from build123d import *

# Parameters (mm, degrees)
BOSS_EXTRUDE1_DEPTH = 1.5875
FILLET1_R           = 2.54
CUT_EXTRUDE1_DEPTH  = 7.62


with BuildPart() as part:
    # Sketch2 → Boss-Extrude1 (new body, symmetric)
    with BuildSketch(Plane.XY):
        with BuildLine():
            add(Edge.make_bspline(
                [(825.5, 263.72872798), (833.004293944, 262.763036085), (840.535916247, 261.846014478), (848.126574562, 260.964164828), (892.90639318, 255.945629274), (937.686211733, 251.779150949), (973.452075064, 248.227669425), (1071.946672141, 239.051054038), (1170.441269319, 229.731506738), (1231.791940344, 224.503945813), (1324.899336146, 216.790627817), (1418.006730935, 209.040117978), (1449.742935921, 206.361809936), (1636.928606778, 190.521130342), (1824.114277635, 175.409157235), (1979.966947376, 164.299650253), (2156.268639429, 150.414433314), (2332.570330468, 133.857216402), (2354.212983157, 131.78508222), (2394.341467798, 127.847039259), (2434.469952439, 123.717187755), (2453.57670361, 121.704562273), (2472.669581058, 119.647220503), (2491.74, 117.547195763)],
                knots=[78.681340958, 78.681340958, 78.681340958, 78.681340958, 78.681340958, 78.681340958, 82.46579272, 82.46579272, 82.46579272, 100.7932901, 100.7932901, 100.7932901, 131.0989539, 131.0989539, 131.0989539, 146.7691983, 146.7691983, 146.7691983, 223.5339586, 223.5339586, 223.5339586, 233.9431167, 233.9431167, 233.9431167, 243.40815085, 243.40815085, 243.40815085, 243.40815085, 243.40815085, 243.40815085], degree=5))
            Line((825.5, 263.72872798), (825.5, 248.364439806))
            add(Edge.make_bspline(
                [(825.5, 248.364439806), (827.20768691, 248.14708351), (833.784664511, 247.321927102), (845.28106727, 245.953419483), (860.086531547, 244.295598067), (879.830703434, 242.186646028), (904.369967092, 239.698279806), (933.571022669, 236.832150625), (962.642718041, 234.023667741), (991.762593943, 231.241975908), (1021.072010315, 228.475862291), (1060.376437315, 224.796956681), (1109.513015577, 220.184378862), (1168.511190361, 214.817071985), (1227.500129793, 209.662054042), (1306.133167947, 203.021178328), (1404.361477105, 194.920725932), (1522.239851071, 184.918066624), (1640.182856491, 175.167007786), (1758.165352567, 165.757639485), (1876.155384769, 156.590937079), (1994.08749188, 147.453250142), (2092.268692061, 139.624216053), (2170.748029042, 133.079656729), (2219.771730977, 128.842227836), (2258.983988247, 125.347211495), (2288.379457536, 122.670854497), (2317.812243116, 119.931729386), (2347.551509172, 117.100365283), (2377.159899727, 114.21011853), (2406.469653851, 111.26896801), (2435.81832606, 108.240091266), (2464.242715806, 105.222889554), (2482.876892709, 103.192325927), (2491.74, 102.214848055)],
                knots=[78.875303138, 78.875303138, 78.875303138, 78.875303138, 79.386176103, 80.841530691, 82.29688528, 83.752239868, 86.662949044, 89.57365822, 92.484367397, 95.395076573, 98.305785749, 101.216494926, 107.037913278, 112.859331631, 118.680749984, 124.502168336, 136.145005042, 147.787841747, 159.430678452, 171.073515158, 182.716351863, 194.359188568, 206.002025273, 211.823443626, 217.644861979, 220.555571155, 223.466280331, 226.376989508, 229.287698684, 232.19840786, 235.109117037, 238.019826213, 240.930535389, 243.57402126, 243.57402126, 243.57402126, 243.57402126], degree=3))
            Line((2491.74, 102.214848055), (2491.74, 117.547195763))
        make_face()
    extrude(amount=BOSS_EXTRUDE1_DEPTH, both=True)

    # Fillet1
    fillet1_edges = [part.edges().sort_by_distance(p)[0] for p in [
        (2491.74, 102.214848055, -0.79375),
        (2491.74, 117.547195763, -0.79375),
        (825.5, 248.364439806, -0.79375),
        (825.5, 263.72872798, 0.79375),
    ]]
    fillet(fillet1_edges, radius=FILLET1_R)

    # Sketch3 → Cut-Extrude1 (cut)
    with BuildSketch(Plane.XY.offset(1.5875)):
        Polygon((1201.641901464, 227.227804562), (1201.641901464, 234.542162162), (821.218059657, 281.929544487), (821.218059657, 218.449722533), (1203.044971141, 207.573021892), (1203.044971141, 212.261982037), (1207.495802024, 221.814984909), (1197.508571749, 218.449722533), align=None)
        Polygon((1554.781712943, 197.53701635), (1561.124210439, 190.02917074), (1551.311808982, 190.02917074), (1557.611128436, 183.063577113), (1557.611128436, 178.064185516), (2509.688563149, 67.607566775), (2509.688563149, 142.671449404), (1554.781712943, 201.416206561), align=None)
    extrude(amount=-CUT_EXTRUDE1_DEPTH, mode=Mode.SUBTRACT)


solid = part.part
Can you work these out from the model? Positions are in its coordinate system, mm. Coordinates: 2 decimals unless noted, no trailing zeros. Answer as CSV lines item,"result". Start each with the question number.
1. Thinking about a two-plate mould opening in Y: for faces 1 (the face through (1554.417, 186.595, 0.022)), 2 (the face through (1380, 205, 1.588)), 3 (the face through (1557.909, 193.836, 0.022)), which applies, +Y half, -Y half, draft (parallel to the pull), parting line (faces both ways), or undercut?
2. If I drill on probe 1 along Y at (x, z) = (1345.5, -0.5); probe 2 along Y at (x, z) = (1225, -1.2), over which ranges is the centre line in solid material (lowest first)? Write a range as [from, to].
3. For pin 1 Ø1 at (x, z) = (1486.5, -0.5) entering from -Y; pin 2 Ø0.5 at (y, z) = (182.5, 0.5) entering from +X, each with a flat end and sliding along its axis, tell me the tip position at first contact or that it passes through.
Output:
1,face 1,"undercut"
1,face 2,"draft"
1,face 3,"+Y half"
2,probe 1,"y = [199.78, 215.07]"
2,probe 2,"y = [209.91, 225.2]"
3,pin 1,"stops at y = 187.92"
3,pin 2,"stops at x = 1557.61"
